from build123d import *

# Parameters (mm, degrees)
BOSS_EXTRUDE3_DEPTH = 10
SKETCH19_R          = 2
SKETCH19_R_2        = 4.05
CUT_EXTRUDE13_DEPTH = 97.545326143
SKETCH24_R          = 1.75
CUT_EXTRUDE17_DEPTH = 10
SKETCH30_W          = 4.5
SKETCH30_H          = 7
SKETCH30_W_2        = 7
SKETCH30_H_2        = 1
BOSS_EXTRUDE4_DEPTH = 5
CUT_EXTRUDE19_DEPTH = 9
CUT_EXTRUDE21_DEPTH = 4
SKETCH31_R          = 1.5
CUT_EXTRUDE24_DEPTH = 97.545326143
SKETCH29_R          = 2
CUT_EXTRUDE23_DEPTH = 2
FILLET2_R           = 0.5
FILLET1_R           = 3


with BuildPart() as part:
    # Sketch17 → Boss-Extrude3 (new body)
    with BuildSketch(Plane(origin=(0, 0, 0), x_dir=(0, 0, -1), z_dir=(1, 0, 0))):
        Polygon((14, -60), (14, -95), (0, -95), (0, 0), (14, 0), (14, -45), align=None)
    extrude(amount=BOSS_EXTRUDE3_DEPTH)

    # Sketch19 → Cut-Extrude13 (cut, through all)
    with BuildSketch(Plane.ZY):
        with Locations((-7, -56)):
            Circle(SKETCH19_R)
        with Locations((-7, -68)):
            Circle(SKETCH19_R_2)
        with Locations((-7, -80)):
            Circle(SKETCH19_R)
    extrude(amount=-CUT_EXTRUDE13_DEPTH, mode=Mode.SUBTRACT)

    # Sketch24 → Cut-Extrude17 (cut)
    with BuildSketch(Plane.ZY):
        with Locations((-10, -5)):
            Circle(SKETCH24_R)
        with Locations((-10, -91)):
            Circle(SKETCH24_R)
    extrude(amount=-CUT_EXTRUDE17_DEPTH, mode=Mode.SUBTRACT)

    # Sketch30 → Boss-Extrude4 (add)
    with BuildSketch(Plane(origin=(10, 0, 0), x_dir=(0, 0, -1), z_dir=(1, 0, 0))):
        with Locations((-2.25, -15)):
            Rectangle(SKETCH30_W, SKETCH30_H)
        with Locations((-2.25, -85)):
            Rectangle(SKETCH30_W, SKETCH30_H)
        with Locations((5, 0.5)):
            Rectangle(SKETCH30_W_2, SKETCH30_H_2)
    extrude(amount=-BOSS_EXTRUDE4_DEPTH)

    # Sketch26 → Cut-Extrude19 (cut)
    with BuildSketch(Plane.ZY):
        with BuildLine():
            Line((-7, -13.35), (7, -13.35))
            ThreePointArc((7, -13.35), (8.65, -15), (7, -16.65))
            Line((7, -16.65), (-7, -16.65))
            ThreePointArc((-7, -16.65), (-8.65, -15), (-7, -13.35))
        make_face()
        with BuildLine():
            Line((-7, -83.35), (7, -83.35))
            ThreePointArc((7, -83.35), (8.65, -85), (7, -86.65))
            Line((7, -86.65), (-7, -86.65))
            ThreePointArc((-7, -86.65), (-8.65, -85), (-7, -83.35))
        make_face()
        with BuildLine():
            Line((-3.35, 8), (-3.35, -8))
            ThreePointArc((-3.35, -8), (-5, -9.65), (-6.65, -8))
            Line((-6.65, -8), (-6.65, 8))
            ThreePointArc((-6.65, 8), (-5, 9.65), (-3.35, 8))
        make_face()
    extrude(amount=-CUT_EXTRUDE19_DEPTH, mode=Mode.SUBTRACT)

    # Sketch27 → Cut-Extrude21 (cut)
    with BuildSketch(Plane.ZY):
        with BuildLine():
            Line((-22.181406925, -44.5), (2.318593075, -44.5))
            ThreePointArc((2.318593075, -44.5), (2.672146466, -44.646446609), (2.818593075, -45))
            Line((2.818593075, -45), (2.818593075, -48))
            ThreePointArc((2.818593075, -48), (2.672146466, -48.353553391), (2.318593075, -48.5))
            Line((2.318593075, -48.5), (-22.181406925, -48.5))
            Line((-22.181406925, -48.5), (-22.181406925, -44.5))
        make_face()
        with BuildLine():
            Line((-22.181406925, -36.5), (2.74769439, -36.5))
            ThreePointArc((2.74769439, -36.5), (2.783233621, -36.501264636), (2.818593075, -36.505052148))
            Line((2.818593075, -36.505052148), (2.818593075, -39.642901183))
            ThreePointArc((2.818593075, -39.642901183), (2.931519183, -40.189011364), (2.468621026, -40.5))
            Line((2.468621026, -40.5), (-22.181406925, -40.5))
            Line((-22.181406925, -40.5), (-22.181406925, -36.5))
        make_face()
    extrude(amount=-CUT_EXTRUDE21_DEPTH, mode=Mode.SUBTRACT)

    # Sketch31 → Cut-Extrude24 (cut, through all)
    with BuildSketch(Plane(origin=(10, 0, 0), x_dir=(0, 0, -1), z_dir=(1, 0, 0))):
        with Locations((0, -90)):
            Circle(SKETCH31_R)
        with Locations((0, -80)):
            Circle(SKETCH31_R)
        with Locations((0, -20)):
            Circle(SKETCH31_R)
        with Locations((0, -10)):
            Circle(SKETCH31_R)
        with Locations((10, 0)):
            Circle(SKETCH31_R)
        Circle(SKETCH31_R)
    extrude(amount=-CUT_EXTRUDE24_DEPTH, mode=Mode.SUBTRACT)

    # Sketch29 → Cut-Extrude23 (cut)
    with BuildSketch(Plane.ZY):
        with Locations((-10, -5)):
            Circle(SKETCH29_R)
        with Locations((-10, -91)):
            Circle(SKETCH29_R)
    extrude(amount=-CUT_EXTRUDE23_DEPTH, mode=Mode.SUBTRACT)

    # Fillet2
    fillet2_edges = [part.edges().sort_by_distance(p)[0] for p in [
        (2, -48.5, -14),
        (2, -44.5, -14),
        (2, -48.5, 0),
        (2, -44.5, 0),
        (5, 0, -14),
        (5, -95, 0),
        (2, -36.5, -14),
        (2, -40.5, -14),
        (2, -36.5, 0),
        (2, -40.5, 0),
        (7.5, 1, -8.5),
        (7, 1, -6.65),
        (7, 1, -3.35),
        (7.5, 1, -1.5),
        (7.5, -81.5, 4.5),
        (7, -83.35, 4.5),
        (7, -86.65, 4.5),
        (7.5, -88.5, 4.5),
        (7.5, -11.5, 4.5),
        (7.5, -18.5, 4.5),
        (7, -13.35, 4.5),
        (7, -16.65, 4.5),
    ]]
    fillet(fillet2_edges, radius=FILLET2_R)

    # Fillet1
    fillet1_edges = [part.edges().sort_by_distance(p)[0] for p in [
        (5, -95, -14),
    ]]
    fillet(fillet1_edges, radius=FILLET1_R)


solid = part.part
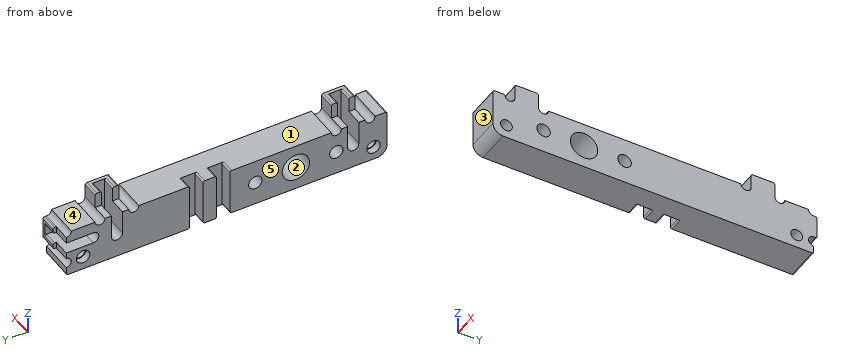
Design review of the part built by this model. Coordinates are the model's own, in mm. Face numbers are marked on the shaded views. A direction names the side the tool comes from. Coordinates: 2 decimals unless noted, no trailing zeros. Order: outer loops, then holes, each group sorted by start corner. A loop starts at its lowest first (then second) coordinate and runs counter-clockwise, first axis right, second up. Notation, with made-up numbers: M 67,36.25 L 77,36.25 A27 ccw 77,67.25 Z; hole C 21.5,-12 d6. An arc over 180 degrees is marked long. Use a Markdown table: item, result.
(1) Add section A-A (z = 1.5). Give the boundary of the cut face in (x, y).
Worked answers:
| item | result |
|---|---|
| outline | M 5,-88.5 L 10,-88.5 L 10,-81.5 L 5,-81.5 L 5,-83.35 L 9,-83.35 L 9,-86.65 L 5,-86.65 Z; M 5,-18.5 L 10,-18.5 L 10,-11.5 L 5,-11.5 L 5,-13.35 L 9,-13.35 L 9,-16.65 L 5,-16.65 Z |
(2) For P1, Ø2, axis at y = -6, z = -9, coming from the -X side; P2, Ø3, axis at y = -56, z = -7, coming from the +X side; P3, Ø0.6, axis at x = 2.5, y = -17.5, coming from the +Z side; P4, Ø3, axis at x = 1, z = -9, coming from the +Y side, all flat-tipped, find the tip position at first contact; note any pin that passes through.
Worked answers:
| item | result |
|---|---|
| P1 | stops at x = 0 |
| P2 | passes through |
| P3 | stops at z = 0 |
| P4 | stops at y = 0 |
(3) Add section C-C (x = 7). Count the separate pieces of the cut face and the enclosed holes in it, then the cut area to 3 significant figures.
Worked answers:
| item | result |
|---|---|
| separate pieces | 1 |
| enclosed holes | 5 |
| area | 1,160 mm2 |
(4) Add section D-D (y = -5). Give the boundary of the cut face in (x, z), then the cut area to 3 significant figures.
Worked answers:
| item | result |
|---|---|
| outline | M 0,-14 L 10,-14 L 10,-11.75 L 2,-11.75 L 2,-12 L 0,-12 Z; M 0,-8 L 2,-8 L 2,-8.25 L 10,-8.25 L 10,0 L 0,0 L 0,-3.35 L 9,-3.35 L 9,-6.65 L 0,-6.65 Z |
| area | 74.3 mm2 |
(5) Add section B-B (y = -80). Give the boundary of the cut face in (x, z).
Worked answers:
| item | result |
|---|---|
| outline | M 0,-14 L 10,-14 L 10,-9 L 0,-9 Z; M 0,-5 L 10,-5 L 10,-1.5 L 0,-1.5 Z |
(6) Draft analysis for pull direction Z (two halves, no side actions). For the marked faces 1, 2 and 3, state which applies: released by +Z, released by -Z, zero draft, split by the parting line, or undercut.
Worked answers:
| item | result |
|---|---|
| face 1 | released by +Z |
| face 2 | undercut |
| face 3 | zero draft |
(7) Wall thickness on probe 1 along Y at (x, z) = (1.25, -2.5); probe 2 along Y at (x, z) = (0.65, -10); probe 3 along Y at (x, z) = (7.5, -7): over which ranges is each line inside the solid? List them lowest first.
Worked answers:
| item | result |
|---|---|
| probe 1 | y = -95 to -86.65, -83.35 to -48.5, -44.5 to -40.5, -36.5 to -16.65, -13.35 to 0 |
| probe 2 | y = -95 to -93, -89 to -70.72, -65.28 to -48.5, -44.5 to -40.5, -36.5 to -7, -3 to -1.5 |
| probe 3 | y = -95 to -86.65, -83.35 to -82, -78 to -72.05, -63.95 to -58, -54 to -16.65, -13.35 to 0.98 |
(8) For the marked faces 4 and 5, list the 3-axis set-ups (+Z, -Z, +X, -X, +Y, -Y) from which the entire face can be reached by the end or side of a thin tool; tool diameter is ignored.
Worked answers:
| item | result |
|---|---|
| face 4 | +Z, +X, -X, +Y |
| face 5 | +Z, -Z, -X, +Y, -Y |
